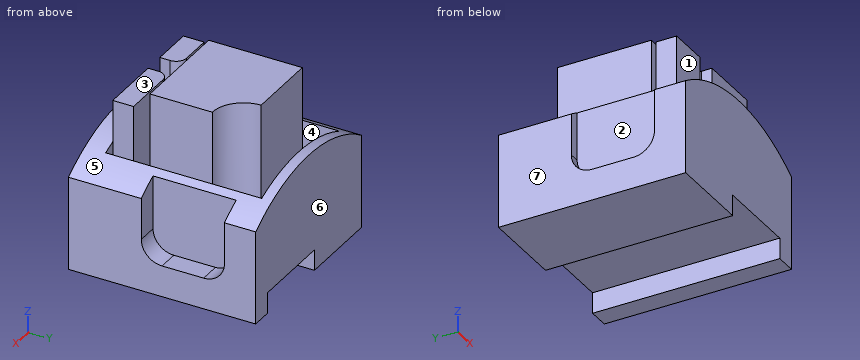
from build123d import *

# Parameters (mm, degrees)
F1_DEPTH  = 90
F3_W      = 60
F3_H      = 75
F4_DEPTH  = 28.8572172234
F6_DEPTH  = 75
F7_W      = 20
F7_H      = 10
F7_W_2    = 30
F8_DEPTH  = 45
F9_R      = 5
F11_DEPTH = 50
F13_W     = 5
F13_H     = 40
F13_W_2   = 10
F14_DEPTH = 65.001
F15_R     = 10


with BuildPart() as f1:
    # F0 (on Front) → F1 (new body)
    with BuildSketch(Plane.XZ):
        with BuildLine():
            Line((0, 45), (0, 0))
            Line((0, 0), (40, 0))
            Line((40, 0), (40, 10))
            Line((40, 10), (80, 10))
            Line((80, 10), (80, 0))
            Line((80, 0), (90, 0))
            Line((90, 0), (90, 45))
            ThreePointArc((90, 45), (45, 58.8562172234), (0, 45))
        make_face()
    extrude(amount=-F1_DEPTH)

    # F3 (on offset) → F4 (cut, through all)
    with BuildSketch(Plane(origin=(0, 0, 30), x_dir=(1, 0, 0), z_dir=(0, 0, -1))):
        with Locations((40, -47.5)):
            Rectangle(F3_W, F3_H)
    extrude(amount=-F4_DEPTH, mode=Mode.SUBTRACT)

    # F5 (on face) → F6 (cut, through all)
    with BuildSketch(Plane.XZ.offset(-85)):
        Polygon((70, 54.8496379912), (70, 30), (76.658440432, 54.8496379912), align=None)
    extrude(amount=F6_DEPTH, mode=Mode.SUBTRACT)

    # F7 (on face) → F8 (join)
    with BuildSketch(Plane.XY.offset(30)):
        with Locations((20, 15)):
            Rectangle(F7_W, F7_H)
        with Locations((55, 15)):
            Rectangle(F7_W_2, F7_H)
    extrude(amount=F8_DEPTH)

    # F9
    f9_edges = [f1.edges().sort_by_distance(p)[0] for p in [
        (40, 20, 52.5),
        (30, 20, 52.5),
    ]]
    fillet(f9_edges, radius=F9_R)

    # F10 (on face) → F11 (join)
    with BuildSketch(Plane.XY.offset(30)):
        with BuildLine():
            Line((50, 70), (15, 70))
            Line((15, 70), (15, 25))
            Line((15, 25), (65, 25))
            Line((65, 25), (65, 55))
            ThreePointArc((65, 55), (54.3933982822, 59.3933982822), (50, 70))
        make_face()
    extrude(amount=F11_DEPTH)

    # F13 (on offset) → F14 (cut, through all)
    with BuildSketch(Plane(origin=(0, 0, 15), x_dir=(1, 0, 0), z_dir=(0, 0, -1))):
        with Locations((2.5, -35)):
            Rectangle(F13_W, F13_H)
        with Locations((85, -55)):
            Rectangle(F13_W_2, F13_H)
    extrude(amount=-F14_DEPTH, mode=Mode.SUBTRACT)

    # F15
    f15_edges = [f1.edges().sort_by_distance(p)[0] for p in [
        (2.5, 55, 15),
        (2.5, 15, 15),
        (85, 35, 15),
        (85, 75, 15),
    ]]
    fillet(f15_edges, radius=F15_R)


solid = f1.part
Build history of the part. All positions in model axes, mm. Face numbers are marked on the shaded views. A direction names the side the tool comes from. Coordinates: 2 decimals unless noted, no trailing zeros. Write each loop counter-clockwise with the first axis right and the second up, starting at its lowest first coordinate (ties: lowest second). Pieces come first, ordered by that corner, then holes. Notation, with made-up numbers: (-16.75, -30) -> (38.25, -30) arc R13 ccw to (38.25, -11) -> close; hole circle Ø3 at (54.5, -12). An arc over 180 degrees is marked (long way). Use CSV: the item, a comma, the result in double quotes. Start each with the question number.
Q1. Flat gauge pins, fed straight in: pin 1 Ø2 at (x, z) = (17.5, 59.5) entering from -Y; pin 2 Ø16.5 at (y, z) = (58, 42.5) entering from +X; pin 3 Ø14.5 at (x, z) = (43.5, 38.5) entering from -Y; pin 4 Ø3 at (y, z) = (16, 66.5) entering from -X. Where does each tip first touch, or does it go through?
Q2. Cut at A-A, the plane z = 67. List the corners of the cut face in (x, y), then the cut area to 3 significant figures.
Q3. Pull direction X, two halves, no side cores. Call the marked faces 4, 5, 6 and 7: released by +X, released by -X, zero draft, split by the parting line, or undercut.
Q4. Drill centre lines: probe 1 along Y at (x, z) = (36.5, 53); probe 2 along X at (y, z) = (14.5, 49); probe 3 along Y at (x, z) = (43, 52). Where is each one in solid material? Low to high.
Q5. Cut at B-B, the plane z = 32. State how many separate pieces and enclosed holes the cut face has, then the cut area to 3 significant figures.
Q6. Cut at C-C, the plane y = 27. List the corners of the cut face in (x, z), then the cut area to 3 significant figures.
Q7. 3-axis set-ups, long thin cutter, end or side, ignore diameter. For the marked faces 1, 2 and 3: which of +Z, -Z, +X, -X, +Y, -Y reach the whole face in a straight line?
Q8. Cut at D-D, the plane x = 52. List the corners of the cut face in (y, z).
Checked values:
1,pin 1,"stops at y = 10"
1,pin 2,"stops at x = 80"
1,pin 3,"stops at y = 0"
1,pin 4,"stops at x = 10"
2,outline,"(10, 10) -> (30, 10) -> (30, 15) arc R5 ccw to (25, 20) -> (10, 20) -> close; (15, 25) -> (65, 25) -> (65, 55) arc R15 cw to (50, 70) -> (15, 70) -> close; (40, 10) -> (70, 10) -> (70, 20) -> (45, 20) arc R5 ccw to (40, 15) -> close"
2,area,"2,560 mm²"
3,face 4,"undercut"
3,face 5,"split by the parting line"
3,face 6,"zero draft"
3,face 7,"released by -X"
4,probe 1,"y = 0 to 10, 25 to 70, 85 to 90"
4,probe 2,"x = 6.53 to 30, 40 to 70, 75.09 to 83.47"
4,probe 3,"y = 0 to 19.58, 25 to 70, 85 to 90"
5,separate pieces,"2"
5,enclosed holes,"1"
5,area,"5,520 mm²"
6,outline,"(0, 0) -> (40, 0) -> (40, 10) -> (80, 10) -> (80, 0) -> (90, 0) -> (90, 45) arc R80 ccw to (76.05, 52.58) -> (70, 30) -> (65, 30) -> (65, 80) -> (15, 80) -> (15, 30) -> (10, 30) -> (10, 50.79) arc R80 ccw to (5, 48.14) -> (5, 15) -> (0, 15) -> close"
6,area,"5,160 mm²"
7,face 1,"+Z, -X, -Y"
7,face 2,"+Z, -X"
7,face 3,"+Z, +X, -X, -Y"
8,outline,"(0, 10) -> (90, 10) -> (90, 58.55) -> (85, 58.55) -> (85, 30) -> (62.52, 30) -> (62.52, 80) -> (25, 80) -> (25, 30) -> (20, 30) -> (20, 75) -> (10, 75) -> (10, 58.55) -> (0, 58.55) -> close"
